Work out the finished part from the listing and answer in its coordinate system (mm). Give positions to 0.01 mm unless a question says otherwise; leave off trailing zeros. Write each loop counter-clockwise with the first axis right and the second up, starting at its lowest first coordinate (ties: lowest second). Pieces come first, ordered by that corner, then holes. Notation, with made-up numbers: (5, -25) - (61, -25) arc R29 ccw to (61, 6) - close; hole circle Ø2 at (42.5, 40.25). An arc over 180 degrees is marked (long way). Write item = value, one per line.
from build123d import *

# Parameters (mm, degrees)
SKETCH1_R           = 2.75
BOSS_EXTRUDE1_DEPTH = 2


with BuildPart() as part:
    # Sketch1 → Boss-Extrude1 (new body)
    with BuildSketch(Plane(origin=(0, 0, 0), x_dir=(0, 0, -1), z_dir=(1, 0, 0))):
        with BuildLine():
            Line((4, 0), (31, 0))
            Line((31, 0), (31, -15))
            ThreePointArc((31, -15), (35, -19), (39, -15))
            Line((39, -15), (39, 0))
            Line((39, 0), (49, 0))
            ThreePointArc((49, 0), (53, 4), (49, 8))
            Line((49, 8), (4, 8))
            ThreePointArc((4, 8), (0, 4), (4, 0))
        make_face()
        with Locations((4, 4)):
            Circle(SKETCH1_R, mode=Mode.SUBTRACT)
        with Locations((35, -15)):
            Circle(SKETCH1_R, mode=Mode.SUBTRACT)
        with Locations((49, 4)):
            Circle(SKETCH1_R, mode=Mode.SUBTRACT)
    extrude(amount=BOSS_EXTRUDE1_DEPTH)


solid = part.part
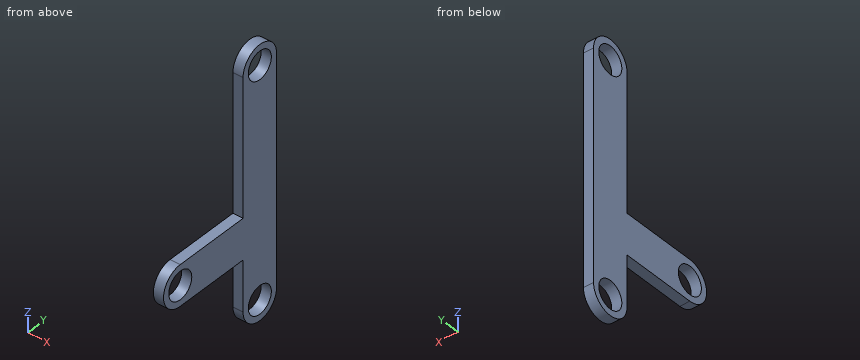
1. Find section C-C, the plane y = 4. Give the vertices of the cut face in (x, z).
Solution:
outline = (0, -53) - (2, -53) - (2, -51.75) - (0, -51.75) - close; (0, -46.25) - (2, -46.25) - (2, -6.75) - (0, -6.75) - close; (0, -1.25) - (2, -1.25) - (2, 0) - (0, 0) - close
2. Given pin 1 (1 mm diameter, centred on x = 0.5, y = 2.5, fed in from -Z); pin 2 (0.6 mm diameter, centred on x = 1, y = -4.5, fed in from +Z); pin 3 (1 mm diameter, centred on x = 1, z = -45, fed in from -Y), each flat-ended and moving along its own axis, determine where each tip first touches the part or whether it passes through.
Solution:
pin_1 = -52.87
pin_2 = -31
pin_3 = 0
3. Find section A-A, the plane x = 0.4. Give the vertices of the cut face in (y, z).
Solution:
outline = (-15, -39) - (0, -39) - (0, -49) arc R4 ccw to (8, -49) - (8, -4) arc R4 ccw to (0, -4) - (0, -31) - (-15, -31) arc R4 ccw to start; hole circle Ø5.5 at (-15, -35); hole circle Ø5.5 at (4, -49); hole circle Ø5.5 at (4, -4)
4. Straight lines are drawn through the part: line 1 (Y direction, x = 0.75, z = -49); line 2 (Z direction, x = 0.2, y = -14.75); line 3 (Y direction, x = 1.85, z = -17). For each, find the intervals that lie inside material, in ascending order.
Solution:
line_1 = 0 to 1.25, 6.75 to 8
line_2 = -39 to -37.74, -32.26 to -31
line_3 = 0 to 8
5. Find section D-D, the plane y = -7.75. Give the vertices of the cut face in (x, z), then the cut area to 3 significant figures.
Solution:
outline = (0, -39) - (2, -39) - (2, -31) - (0, -31) - close
area = 16.0 mm^2
6. Find section B-B, the plane z = -35. Give the vertices of the cut face in (x, y), then the cut area to 3 significant figures.
Solution:
outline = (0, -19) - (2, -19) - (2, -17.75) - (0, -17.75) - close; (0, -12.25) - (2, -12.25) - (2, 8) - (0, 8) - close
area = 43.0 mm^2
